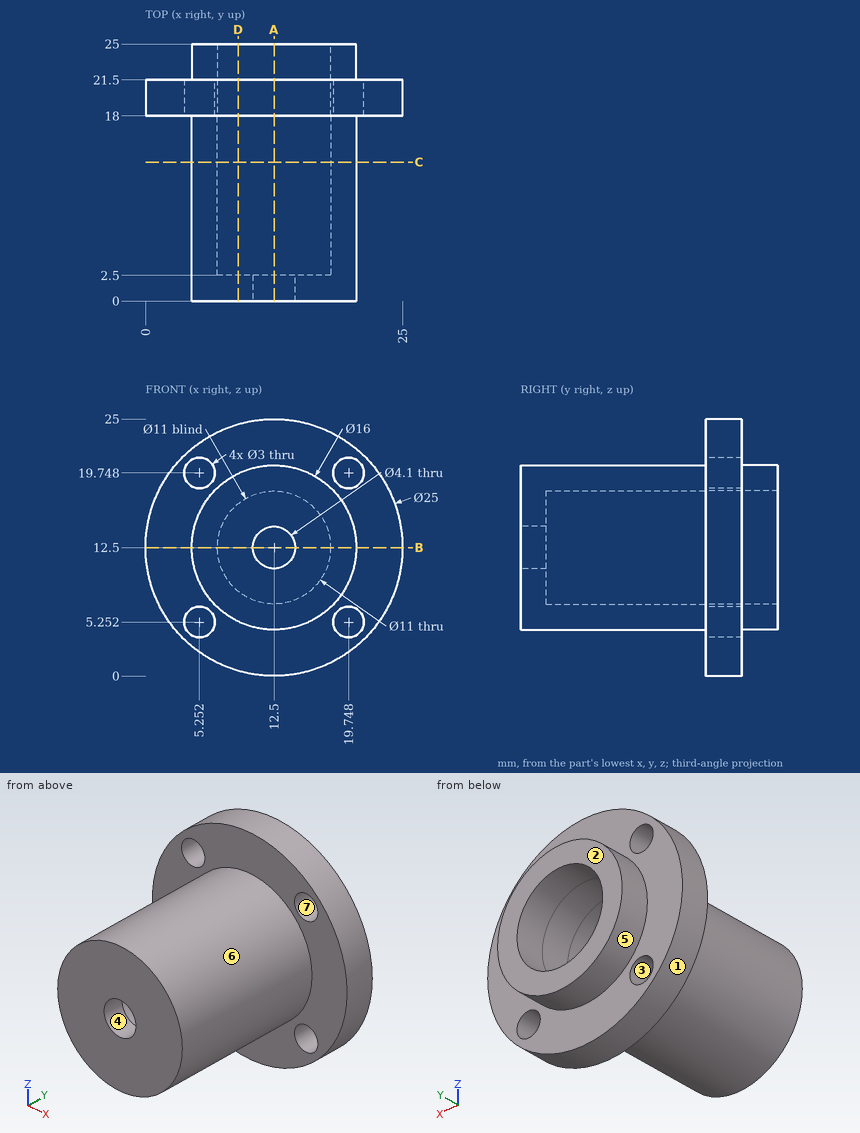
Print and shaded views of the part. All mm, measured from the part's lowest x, y and z. A direction names the side the tool comes from. Round coordinates to 2 decimals unless told otherwise and drop trailing zeros. Loops run counter-clockwise (first coordinate to the right, second up) from the corner with the lowest first, then second, coordinate; pieces in that order, holes last. Notation, with made-up numbers: (84, 55) -> (104, 55) arc R19 ccw to (104, 91) -> close; hole circle Ø4 at (13, 11.25). An arc over 180 degrees is marked (long way). Use CSV: the item, a comma, the result in double quotes. Start each with the question number.
1) Cut at C-C, the plane y = 13.5. Write the cut outline in (x, z).
2) Cut at A-A, the plane x = 12.5. Write the cut outline in (y, z), plus the area to 3 significant figures.
3) Cut at D-D, the plane x = 9. Write the cut outline in (y, z), plus the area to 3 significant figures.
4) Pull direction X, two halves, no side cores. Call the marked faces 1, 2, 3 and 4: +X half, -X half, draft (parallel to the pull), parting line (faces both ways), or undercut.
5) Drop flat-ended pins along their axis: P1, Ø6.5, axis at x = 12.5, z = 12.5, coming from the +Y side; P2, Ø5.5, axis at x = 11, z = 15, coming from the +Y side; P3, Ø4, axis at y = 12, z = 19.5, coming from the -X side (1 decimal); P4, Ø6, axis at x = 20, y = 3.5, coming from the +Z side. Give the stop position or say it passes through.
6) Cut at B-B, the plane z = 12.5. Write the cut outline in (x, y).
7) Wall check: L1, parallel to Z at x = 12.5, y = 22.4; L2, parallel to Z at x = 12.5, y = 1. Give the ranges that are in metal, low to high. Write a range as [from, to].
8) Which spindle directions (+Z, -Z, +X, -X, +Y, -Y) get a long thin tool onto all of the face, cutting with end or side? Do the marked faces 5, 6 and 7. Say none if no direction does.
Determined:
1,outline,"circle Ø16 at (12.5, 12.5); hole circle Ø11 at (12.5, 12.5)"
2,outline,"(0, 4.5) -> (18, 4.5) -> (18, 0) -> (21.5, 0) -> (21.5, 4.5) -> (25, 4.5) -> (25, 7) -> (2.5, 7) -> (2.5, 10.45) -> (0, 10.45) -> close; (0, 14.55) -> (2.5, 14.55) -> (2.5, 18) -> (25, 18) -> (25, 20.5) -> (21.5, 20.5) -> (21.5, 25) -> (18, 25) -> (18, 20.5) -> (0, 20.5) -> close"
2,area,"174 mm2"
3,outline,"(0, 5.31) -> (18, 5.31) -> (18, 0.5) -> (21.5, 0.5) -> (21.5, 5.31) -> (25, 5.31) -> (25, 8.26) -> (2.5, 8.26) -> (2.5, 16.74) -> (25, 16.74) -> (25, 19.69) -> (21.5, 19.69) -> (21.5, 24.5) -> (18, 24.5) -> (18, 19.69) -> (0, 19.69) -> close"
3,area,"202 mm2"
4,face 1,"parting line"
4,face 2,"draft"
4,face 3,"undercut"
4,face 4,"undercut"
5,P1,"stops at y = 2.5"
5,P2,"stops at y = 25"
5,P3,"stops at x = 6.3"
5,P4,"stops at z = 19.11"
6,outline,"(0, 18) -> (4.5, 18) -> (4.5, 0) -> (10.45, 0) -> (10.45, 2.5) -> (7, 2.5) -> (7, 25) -> (4.5, 25) -> (4.5, 21.5) -> (0, 21.5) -> close; (14.55, 0) -> (20.5, 0) -> (20.5, 18) -> (25, 18) -> (25, 21.5) -> (20.5, 21.5) -> (20.5, 25) -> (18, 25) -> (18, 2.5) -> (14.55, 2.5) -> close"
7,L1,"z = [4.5, 7], [18, 20.5]"
7,L2,"z = [4.5, 10.45], [14.55, 20.5]"
8,face 5,"+Y"
8,face 6,"-Y"
8,face 7,"+Y, -Y"
